Check sheet for the modelled part. Datum: model origin and axes. Units: mm. Face numbers are marked on the shaded views. Coordinates: 2 decimals unless noted, no trailing zeros. Write each loop counter-clockwise with the first axis right and the second up, starting at its lowest first coordinate (ties: lowest second). Pieces come first, ordered by that corner, then holes. Notation, with made-up numbers: (74, 41) -> (106, 41) arc R30 ccw to (106, 72) -> close; hole circle Ø5 at (64.5, 69.25). An arc over 180 degrees is marked (long way). One line per item, written item: value. Start each with the question number.
1) Gauge pin test, flat ends, axial feed: P1, Ø6.5, axis at x = 0, y = 15, coming from the +Z side (3 decimals); P2, Ø3, axis at y = 21, z = 6.5, coming from the +X side; P3, Ø1.5, axis at x = 9, z = 2, coming from the +Y side; P4, Ø6, axis at y = 4.5, z = 17, coming from the -X side. Record the tip position at first contact, or that the pin passes through.
2) Sectioned sample at A-A on y = -7.5. Enter the section's corners in (x, z), plus the area to 3 significant figures.
3) Scan lines: line 1 along Y through (x, z) = (2.5, 7.75); line 2 along X through (y, z) = (-8.5, 3.75); line 3 along X through (y, z) = (13, 16). Record each from-to range of solid material in increasing order. Write a range as [from, to].
4) Sectioned sample at D-D on x = -1. Enter the section's corners in (y, z), plus the area to 3 significant figures.
5) Sectioned sample at B-B on z = 7. Enter the section's corners in (x, y) (3 decimals), plus the area to 3 significant figures.
6) Draft check along Y on the marked faces 1, 2 and 3. Enter one of: +Y half, -Y half, draft (parallel to the pull), parting line (faces both ways), or undercut.
7) Sectioned sample at C-C on y = 0. Enter the section's corners in (x, z) (3 decimals), plus the area to 3 significant figures.
```python
from build123d import *

# Parameters (mm, degrees)
F0_R     = 4.15
F0_R_2   = 4.1
F0_R_3   = 4.125
F0_R_4   = 4.05
F1_DEPTH = 20
F2_R     = 2


with BuildPart() as f1:
    # F0 (on Top) → F1 (new body)
    with BuildSketch(Plane.XY):
        with BuildLine():
            ThreePointArc((0, 25), (-5, 23.660254), (-8.660254, 20))
            Line((-8.660254, 20), (-21.650635, -2.5))
            ThreePointArc((-21.650635, -2.5), (-21.650635, -12.5), (-12.990381, -17.5))
            Line((-12.990381, -17.5), (12.990381, -17.5))
            ThreePointArc((12.990381, -17.5), (21.650635, -12.5), (21.650635, -2.5))
            Line((21.650635, -2.5), (8.660254, 20))
            ThreePointArc((8.660254, 20), (5, 23.660254), (0, 25))
        make_face()
        with Locations((-12.990381, -7.5)):
            Circle(F0_R, mode=Mode.SUBTRACT)
        with Locations((12.990381, -7.5)):
            Circle(F0_R_2, mode=Mode.SUBTRACT)
        Circle(F0_R_3, mode=Mode.SUBTRACT)
        with Locations((0, 15)):
            Circle(F0_R_4, mode=Mode.SUBTRACT)
        with BuildLine():
            Line((0, 35), (-8.660254, 20))
            ThreePointArc((-8.660254, 20), (-5, 23.660254), (0, 25))
            Line((0, 25), (0, 35))
        make_face()
    extrude(amount=F1_DEPTH)

    # F2
    f2_edges = [f1.edges().sort_by_distance(p)[0] for p in [
        (0, 35, 10),
    ]]
    fillet(f2_edges, radius=F2_R)


solid = f1.part
```
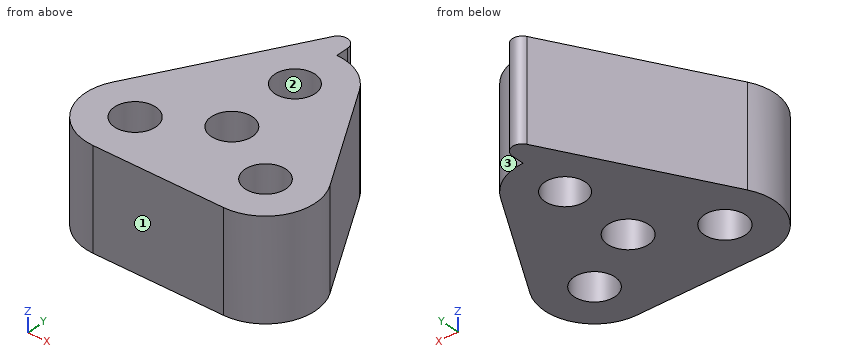
Answers:
1. P1: passes through
1. P2: stops at x = 8.95
1. P3: stops at y = 20.65
1. P4: stops at x = -19.34
2. outline: (-22.99, 0) -> (-17.14, 0) -> (-17.14, 20) -> (-22.99, 20) -> close; (-8.84, 0) -> (8.89, 0) -> (8.89, 20) -> (-8.84, 20) -> close; (17.09, 0) -> (22.99, 0) -> (22.99, 20) -> (17.09, 20) -> close
2. area: 590 mm2
3. line 1: y = [-17.5, -3.28], [3.28, 11.81], [18.19, 24.68]
3. line 2: x = [-22.94, -17.02], [-8.96, 9.01], [16.97, 22.94]
3. line 3: x = [-12.7, -3.52], [3.52, 12.7]
4. outline: (-17.5, 0) -> (-4, 0) -> (-4, 20) -> (-17.5, 20) -> close; (4, 0) -> (11.08, 0) -> (11.08, 20) -> (4, 20) -> close; (18.92, 0) -> (29.27, 0) -> (29.27, 20) -> (18.92, 20) -> close
4. area: 618 mm2
5. outline: (-21.651, -2.5) arc R10 ccw to (-12.99, -17.5) -> (12.99, -17.5) arc R10 ccw to (21.651, -2.5) -> (8.66, 20) arc R10 ccw to (0, 25) -> (0, 27.536) arc R2 ccw to (-3.732, 28.536) -> close; hole circle Ø8.3 at (-12.99, -7.5); hole circle Ø8.25 at (0, 0); hole circle Ø8.1 at (0, 15); hole circle Ø8.2 at (12.99, -7.5)
5. area: 1,200 mm2
6. face 1: -Y half
6. face 2: undercut
6. face 3: +Y half
7. outline: (-20.207, 0) -> (-4.125, 0) -> (-4.125, 20) -> (-20.207, 20) -> close; (4.125, 0) -> (20.207, 0) -> (20.207, 20) -> (4.125, 20) -> close
7. area: 643 mm2
